```python
from build123d import *

# Parameters (mm, degrees)
F0_R      = 18.9595405406
F1_DEPTH  = 152.4
F2_R      = 18.9595405406
F3_DEPTH  = 76.2
F3_TAPER  = 15
F4_W      = 53.2747134566
F4_H      = 4.5048468746
F5_DEPTH  = 50.8
F9_COUNT  = 8
F9_ANGLE  = 210
F10_R     = 13.3778367219
F11_DEPTH = 151.692


with BuildPart() as f1:
    # F0 (on Top) → F1 (new body)
    with BuildSketch(Plane.XY):
        Circle(F0_R)
    extrude(amount=F1_DEPTH)

    # F2 (on face) → F3 (join)
    with BuildSketch(Plane.XY.offset(152.4)):
        Circle(F2_R)
    extrude(amount=F3_DEPTH, taper=F3_TAPER)

    # F4 (on face) → F5 (join)
    with BuildSketch(Plane(origin=(0, 0, 0), x_dir=(1, 0, 0), z_dir=(0, 0, -1))):
        Rectangle(F4_W, F4_H)
    extrude(amount=-F5_DEPTH)

    # F6 (on Front) → F7 (revolve, cut)
    with BuildSketch(Plane.XZ):
        Polygon((-27.585586533, 0), (-21.0148207843, 54.1184917092), (-34.3035459518, 55.4788671434), align=None)
    revolve(axis=Axis((0, 0, -8.6749633774), (0, 0, -1)), mode=Mode.SUBTRACT)

    # F9: F1 ×8 about axis
    f9_axis = Axis((0, 0, -6.7568952218), (0, 0, -1))


with BuildPart() as f1_1:
    add(f1.part)
    for i in range(1, F9_COUNT):
        add(f1.part.rotate(f9_axis, i * F9_ANGLE / (F9_COUNT - 1)))

    # F10 (on face) → F11 (cut)
    with BuildSketch(Plane(origin=(0, 0, 0), x_dir=(1, 0, 0), z_dir=(0, 0, -1))):
        Circle(F10_R)
    extrude(amount=-F11_DEPTH, mode=Mode.SUBTRACT)


solid = f1_1.part
```
Work out the finished part from the listing and answer in its coordinate system (mm). A direction names the side the tool comes from. Give positions to 0.01 mm unless a question says otherwise; leave off trailing zeros. Order: outer loops, then holes, each group sorted by start corner. A loop starts at its lowest first (then second) coordinate and runs counter-clockwise, first axis right, second up. Notation, with made-up numbers: (11, 61.25) - (38, 61.25) arc R18 ccw to (38, 72.25) - close; hole circle Ø11 at (5.5, 81). An arc over 180 degrees is marked (long way). One line per item, written item: value. Start each with the question number.
1. For a pull along Y with two mould halves and no side action, classify faces 5 (the face through (8.915, 2.808, 188.274)), 6 (the face through (-10.616, 8.14, 74.784)), 7 (the face through (17, 10, 50.8)) as released by +Y, released by -Y, zero draft, split by the parting line, or undercut.
2. Consider line 1 (Y direction, x = 0, z = 105); line 2 (Y direction, x = 11.5, z = 32.5). Determine where each line is inside the solid, lowest interval first.
3. Section A-A, the plane z = 174.5 is taken. Write down the section's boundary in (x, y).
4. Which of the six approach directions +Z, -Z, +X, -X, +Y, -Y give full straight-line access (tool end or side, diameter ignored) to faces 1 (the face through (-10, 17, 50.8)), 2 (the face through (-17, -10, 50.8)), 3 (the face through (-8.95, -20.01, 19.4)), 4 (the face through (20.01, -8.95, 19.4))?
5. Each of these flat-tipped pins is pushed along its axis until it touches: pin 1 Ø2 at (x, z) = (-14.5, 120.5) entering from -Y; pin 2 Ø1.5 at (y, z) = (13.5, 45.5) entering from -X; pin 3 Ø8 at (x, y) = (5.5, -2.5) entering from -Z. Where does it stop, or does it pass through?
Filled sheet:
1. face 5: split by the parting line
1. face 6: undercut
1. face 7: zero draft
2. line 1: -18.96 to -13.38, 13.38 to 18.96
2. line 2: -20.65 to -15.41, -15.07 to -6.83, 6.83 to 15.07, 15.41 to 20.65
3. outline: circle Ø26.08 at (0, 0)
4. face 1: +Z, -X, +Y
4. face 2: +Z, -X, -Y
4. face 3: +Z, -Z, -Y
4. face 4: +Z, -Z, +X
5. pin 1: y = -13.31
5. pin 2: x = -18.02
5. pin 3: z = 151.69
